For this review, take the finished solid that the model builds, in its own axes (mm). Coordinates: 2 decimals unless noted, no trailing zeros. Write each loop counter-clockwise with the first axis right and the second up, starting at its lowest first coordinate (ties: lowest second). Pieces come first, ordered by that corner, then holes.
Autodesk Inventor part; units mm, degrees
ref_plane "YZ Plane" through (0, 0, 0) normal (1, 0, 0) x (0, 1, 0)
ref_plane "XZ Plane" through (0, 0, 0) normal (0, 1, 0) x (-1, 0, 0)
ref_plane "XY Plane" through (0, 0, 0) normal (0, 0, 1) x (1, 0, 0)
sketch "Sketch1" plane through (0, 0, 0) normal (0, 1, 0) x (-1, 0, 0)
  line L0 (0, 0) -> (-431.8, 0)
  line L1 (-431.8, 0) -> (-431.8, -431.8)
  line L2 (-431.8, -431.8) -> (0, -431.8)
  line L3 (0, -431.8) -> (0, 0)
  dimension "d0" = 431.8
  dimension "d1" = 431.8
extrude "Extrusion1" add sketch "Sketch1" along normal blind 3.175
sketch "Sketch2" plane through (0, 3.175, 0) normal (0, 1, 0) x (1, 0, 0)
  line L0 (0, 431.8) -> (0, 0)
  line L1 (431.8, 0) -> (431.8, 431.8)
  circle A0 centre (386.08, 64.77) radius 6.35
  circle A1 centre (332.74, 64.77) radius 6.35
  circle A2 centre (279.4, 64.77) radius 6.35
  circle A3 centre (226.06, 64.77) radius 6.35
  circle A4 centre (172.72, 64.77) radius 6.35
  circle A5 centre (28.43, 92.2674) radius 1.5
  circle A6 centre (121.43, 92.2674) radius 1.5
  circle A7 centre (28.43, 37.2726) radius 1.5
  circle A8 centre (121.43, 37.2726) radius 1.5
  line L2 (26.43, 84.77) -> (123.43, 84.77)
  line L3 (123.43, 84.77) -> (123.43, 44.77)
  line L4 (123.43, 44.77) -> (26.43, 44.77)
  line L5 (26.43, 44.77) -> (26.43, 84.77)
  dimension "d14" = 12.7
  dimension "d15" = 12.7
  dimension "d16" = 12.7
  dimension "d17" = 12.7
  dimension "d18" = 12.7
extrude "Extrusion2" cut sketch "Sketch2" against normal blind 25.4
sketch "Sketch3" plane through (0, 3.175, 0) normal (0, 1, 0) x (1, 0, 0)
  line L0 (0, 431.8) -> (0, 0)
  line L1 (431.8, 0) -> (431.8, 431.8)
  circle A0 centre (88.9, 424.18) radius 2.54
  circle A1 centre (115.316, 424.18) radius 2.54
  circle A2 centre (316.484, 424.18) radius 2.54
  circle A3 centre (342.9, 424.18) radius 2.54
  line L2 (431.8, 431.8) -> (431.8, 424.18)
extrude "Extrusion3" cut sketch "Sketch3" along normal blind 25.4 and the other way blind 12.7
sketch "Sketch4" plane through (0, 0, 0) normal (0, -1, 0) x (1, 0, 0)
  circle A0 centre (386.08, -64.77) radius 6.35
  circle A1 centre (386.08, -64.77) radius 6.858
  circle A2 centre (172.72, -64.77) radius 6.35
  circle A3 centre (172.72, -64.77) radius 6.858
  circle A4 centre (226.06, -64.77) radius 6.35
  circle A5 centre (226.06, -64.77) radius 6.858
  circle A6 centre (279.4, -64.77) radius 6.35
  circle A7 centre (279.4, -64.77) radius 6.858
  circle A8 centre (332.74, -64.77) radius 6.35
  circle A9 centre (332.74, -64.77) radius 6.858
  point P0 (0, 0)
  dimension "d50" = 13.716
  dimension "d51" = 13.716
  dimension "d52" = 13.716
  dimension "d53" = 13.716
  dimension "d54" = 13.716
extrude "Extrusion4" cut sketch "Sketch4" against normal blind 4.351 contours A0 | A1 | A2 | A3 | A4 | A5 | A6 | A7 | A8 | A9
sketch "Sketch6" plane through (0, 3.175, 0) normal (0, 1, 0) x (1, 0, 0)
  line L0 (431.8, 0) -> (431.8, 431.8)
  line L1 (0, 431.8) -> (431.8, 431.8)
  line L2 (431.8, 431.8) -> (431.8, 114.3)
  line L3 (431.8, 114.3) -> (0, 114.3)
  line L4 (0, 114.3) -> (0, 431.8)
  line L5 (0, 114.3) -> (431.8, 114.3)
  line L6 (431.8, 114.3) -> (431.8, 12.7)
  line L7 (431.8, 12.7) -> (0, 12.7)
  line L8 (0, 12.7) -> (0, 114.3)
  line L9 (431.8, 0) -> (0, 0)
  line L10 (0, 0) -> (0, 12.7)
  line L11 (0, 12.7) -> (431.8, 12.7)
  line L12 (431.8, 12.7) -> (431.8, 0)
  dimension "d68" = 317.5
  dimension "d69" = 101.6
extrude "Extrusion6" cut sketch "Sketch6" against normal blind 25.4 contours L9 L10 L7 L0 | L3 L4 L1 L0
properties part number "220307 Lid Part B"
Q1. Add section D-D (y = 1.25). Give the number of separate pieces and of enclosed holes in the cut face, then the cut area to 3 significant figures.
Ans:
separate pieces: 1
enclosed holes: 10
area: 39,200 mm2
Q2. Add section B-B (x = 386.08). State the section outline as (y, z) points (3 decimals), then the cut area to 3 significant figures.
Ans:
outline: (0, -114.3) - (3.175, -114.3) - (3.175, -71.628) - (0, -71.628) - close; (0, -57.912) - (3.175, -57.912) - (3.175, -12.7) - (0, -12.7) - close
area: 279 mm2
Q3. Clearance check with a flat-ended pin moving along its axis: pin 1 Ø8 at (x, z) = (226.06, -64.77) entering from -Y (3 decimals). State where the tip first meets the part, or that it passes through.
Ans:
pin 1: passes through
Q4. Add section C-C (x = 90). State the section outline as (y, z) points (3 decimals), then the cut area to 3 significant figures.
Ans:
outline: (0, -114.3) - (3.175, -114.3) - (3.175, -84.77) - (0, -84.77) - close; (0, -44.77) - (3.175, -44.77) - (3.175, -12.7) - (0, -12.7) - close
area: 196 mm2
Q5. Draft analysis for pull direction X (two halves, no side actions). For faces 1 (the flat face through (219, 3.175, -63)), 2 (the cylindrical face through (179.26, 1.57, -62.71)), state which applies: +X half, -X half, draft (parallel to the pull), parting line (faces both ways), or undercut.
Ans:
face 1: draft
face 2: undercut
Q6. For probe 1 along Z at (x, y) = (121.43, 1.85); probe 2 along Z at (x, y) = (51.5, 2.55); probe 3 along X at (y, z) = (1.35, -74.5), list the stretches that pass through material, from the lowest coordinate up.
Ans:
probe 1: z = -114.3 to -93.77, -90.77 to -84.77, -44.77 to -38.77, -35.77 to -12.7
probe 2: z = -114.3 to -84.77, -44.77 to -12.7
probe 3: x = 0 to 26.43, 123.43 to 431.8
Q7. Add section A-A (z = -64.77). State the section outline as (x, y) points (3 decimals), then the cut area to 3 significant figures.
Ans:
outline: (0, 0) - (26.43, 0) - (26.43, 3.175) - (0, 3.175) - close; (123.43, 0) - (165.862, 0) - (165.862, 3.175) - (123.43, 3.175) - close; (179.578, 0) - (219.202, 0) - (219.202, 3.175) - (179.578, 3.175) - close; (232.918, 0) - (272.542, 0) - (272.542, 3.175) - (232.918, 3.175) - close; (286.258, 0) - (325.882, 0) - (325.882, 3.175) - (286.258, 3.175) - close; (339.598, 0) - (379.222, 0) - (379.222, 3.175) - (339.598, 3.175) - close; (392.938, 0) - (431.8, 0) - (431.8, 3.175) - (392.938, 3.175) - close
area: 845 mm2
